The listing builds one solid part. Answer for the finished solid, in the listing's coordinates (mm). A direction names the side the tool comes from. Round coordinates to 2 decimals unless told otherwise and drop trailing zeros. Loops run counter-clockwise (first coordinate to the right, second up) from the corner with the lowest first, then second, coordinate; pieces in that order, holes last. Notation, with made-up numbers: M 20.5,32 L 59.5,32 A24 ccw 59.5,71 Z; hole C 15.25,-20 d5. An arc over 180 degrees is marked long. Put each result on its own line as item: value. Start each with the question number.
(1) Which of the six approach directions +Z, -Z, +X, -X, +Y, -Y give full straight-line access (tool end or side, diameter ignored) to faces 4 (the face through (9, 25, 0)), 5 (the face through (9, 22, 0))?
(2) Straight lines are drawn through the part: line 1 (Z direction, x = -275, y = -5.5); line 2 (Y direction, x = -299, z = -5.25); line 3 (Y direction, x = -550.5, z = 11.25). For each, find the intervals that lie inside material, in ascending order.
(3) Determine the mould class of faces 1 (the face through (9, 0, -12)), 2 (the face through (9, 0, -15)), 3 (the face through (9, -25, 0)) for opening direction Y: released by +Y, released by -Y, zero draft, split by the parting line, or undercut.
(4) Section C-C, the plane z = -0.25 is taken. Determine the outline of the cut face in (x, y).
(5) A flat-ended cylindrical pin translates along its axis: P1, Ø8, axis at y = 10, z = 10.5, coming from the -X side. Find the tip coordinate at first contact, or state that the pin passes through.
(6) Section A-A, the plane y = 4 is taken. Determine the outline of the cut face in (x, z).
(7) Section B-B, the plane x = -172 is taken. Determine the outline of the cut face in (y, z), then the cut area to 3 significant figures.
```python
from build123d import *

# Parameters (mm, degrees)
F0_W     = 50
F0_H     = 30
F0_W_2   = 44
F0_H_2   = 24
F1_DEPTH = 660
F2_R     = 1.5
F3_R     = 4.5


with BuildPart() as f1:
    # F0 (on Right) → F1 (new body, symmetric)
    with BuildSketch(Plane.YZ):
        Rectangle(F0_W, F0_H)
        Rectangle(F0_W_2, F0_H_2, mode=Mode.SUBTRACT)
    extrude(amount=F1_DEPTH, both=True)

    # F2
    f2_edges = [f1.edges().sort_by_distance(p)[0] for p in [
        (0, -22, -12),
        (0, -22, 12),
        (0, 22, -12),
        (0, 22, 12),
    ]]
    fillet(f2_edges, radius=F2_R)

    # F3
    f3_edges = [f1.edges().sort_by_distance(p)[0] for p in [
        (0, -25, 15),
        (0, -25, -15),
        (0, 25, -15),
        (0, 25, 15),
    ]]
    fillet(f3_edges, radius=F3_R)


solid = f1.part
```
Recorded:
1. face 4: +Z, -Z, +X, -X, +Y
1. face 5: +X, -X
2. line 1: z = -15 to -12, 12 to 15
2. line 2: y = -25 to -22, 22 to 25
2. line 3: y = -24.94 to -21.8, 21.8 to 24.94
3. face 1: undercut
3. face 2: zero draft
3. face 3: released by -Y
4. outline: M -660,-25 L 660,-25 L 660,-22 L -660,-22 Z; M -660,22 L 660,22 L 660,25 L -660,25 Z
5. P1: stops at x = -660
6. outline: M -660,-15 L 660,-15 L 660,-12 L -660,-12 Z; M -660,12 L 660,12 L 660,15 L -660,15 Z
7. outline: M -25,-10.5 A4.5 ccw -20.5,-15 L 20.5,-15 A4.5 ccw 25,-10.5 L 25,10.5 A4.5 ccw 20.5,15 L -20.5,15 A4.5 ccw -25,10.5 Z; hole M -22,-10.5 A1.5 ccw -20.5,-12 L 20.5,-12 A1.5 ccw 22,-10.5 L 22,10.5 A1.5 ccw 20.5,12 L -20.5,12 A1.5 ccw -22,10.5 Z
7. area: 429 mm²
